Answer from the drawing. Dimensions are ordinates in mm from the lowest x, y and z of the part. A direction names the side the tool comes from. Give positions to 0.01 mm unless a question says otherwise; leave off trailing zeros. Write each loop counter-clockwise with the first axis right and the second up, starting at its lowest first coordinate (ties: lowest second). Pieces come first, ordered by that corner, then holes.
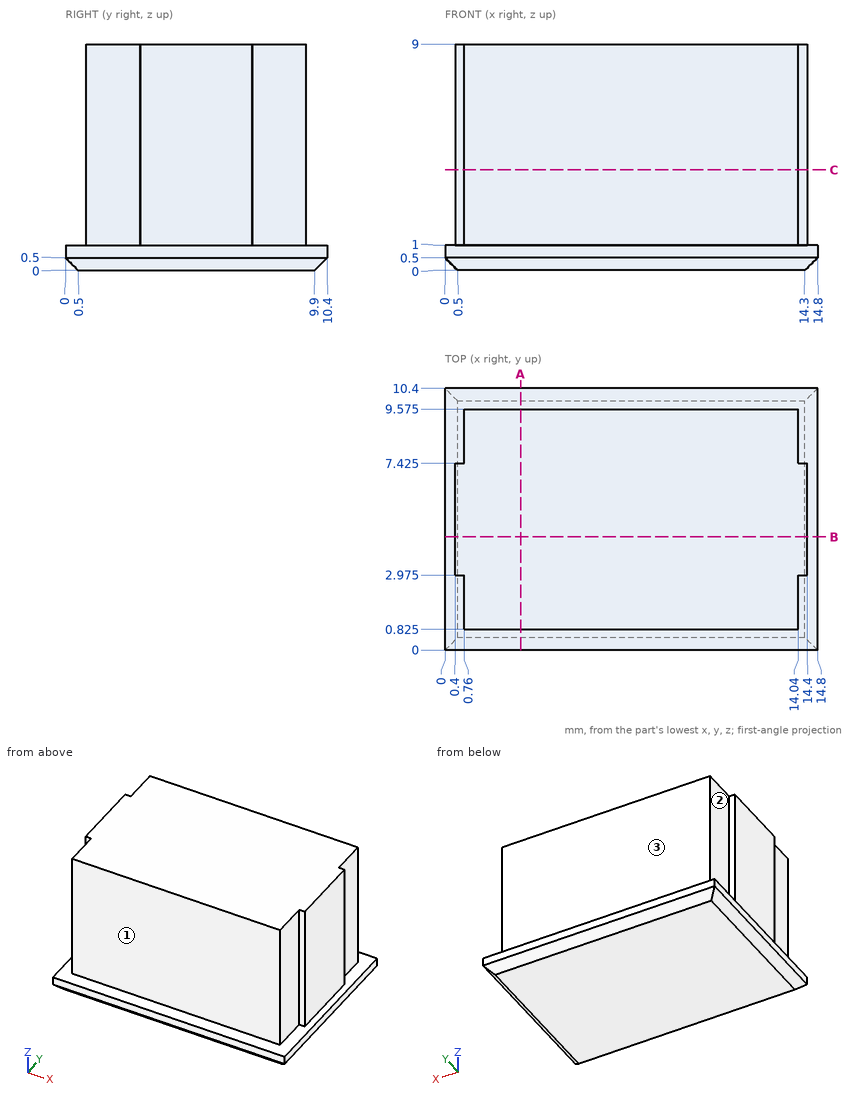
Item 1: A cutting plane is placed at C-C, the plane z = 4. Give the vertices of the cut face in (x, y) (3 decimals), plus the area to 3 significant figures.
Conclusion:
outline: (0.4, 2.975) - (0.76, 2.975) - (0.76, 0.825) - (14.04, 0.825) - (14.04, 2.975) - (14.4, 2.975) - (14.4, 7.425) - (14.04, 7.425) - (14.04, 9.575) - (0.76, 9.575) - (0.76, 7.425) - (0.4, 7.425) - close
area: 119 mm2
Item 2: Each of these flat-tipped pins is pushed along its axis until it touches: P1, Ø1.1, axis at y = 1.5, z = 5.5, coming from the +X side; P2, Ø2, axis at x = 9, z = 7, coming from the +Y side (3 decimals); P3, Ø5, axis at y = 2, z = 7, coming from the -X side. Where does it stop, or does it pass through?
Conclusion:
P1: stops at x = 14.04
P2: stops at y = 9.575
P3: stops at x = 0.4
Item 3: Consider probe 1 along Y at (x, z) = (2.5, 3.5) (3 decimals); probe 2 along X at (y, z) = (7, 6.5); probe 3 along X at (y, z) = (8.5, 5.75). Determine where each line is inside the solid, lowest interval first.
Conclusion:
probe 1: y = 0.825 to 9.575
probe 2: x = 0.4 to 14.4
probe 3: x = 0.76 to 14.04
Item 4: Which of the six approach directions +Z, -Z, +X, -X, +Y, -Y give full straight-line access (tool end or side, diameter ignored) to the marked faces 1, 2 and 3?
Conclusion:
face 1: +Z, +X, -X, -Y
face 2: +Z, -X, +Y
face 3: +Z, +X, -X, +Y
Item 5: A cutting plane is placed at A-A, the plane x = 3. Give the vertices of the cut face in (y, z) (3 decimals).
Conclusion:
outline: (0, 0.5) - (0.5, 0) - (9.9, 0) - (10.4, 0.5) - (10.4, 1) - (9.575, 1) - (9.575, 9) - (0.825, 9) - (0.825, 1) - (0, 1) - close
Item 6: A cutting plane is placed at B-B, the plane y = 4.5. Give the vertices of the cut face in (x, z), plus the area to 3 significant figures.
Conclusion:
outline: (0, 0.5) - (0.5, 0) - (14.3, 0) - (14.8, 0.5) - (14.8, 1) - (14.4, 1) - (14.4, 9) - (0.4, 9) - (0.4, 1) - (0, 1) - close
area: 127 mm2
